Design review of the part built by this model. Coordinates are the model's own, in mm. Face numbers are marked on the shaded views. A direction names the side the tool comes from. Give positions to 0.01 mm unless a question says otherwise; leave off trailing zeros. Loops run counter-clockwise (first coordinate to the right, second up) from the corner with the lowest first, then second, coordinate; pieces in that order, holes last.
from build123d import *

# Parameters (mm, degrees)
EXTRUDE_2_DEPTH       = 5
SKETCH_3_R            = 8
EXTRUDE_3_DEPTH       = 5
SKETCH_4_W            = 60
SKETCH_4_H            = 40
EXTRUDE_4_DEPTH       = 50
SKETCH_5_W            = 70
SKETCH_5_H            = 70
EXTRUDE_5_DEPTH       = 30
SKETCH_6_R            = 2.5
EXTRUDE_6_DEPTH       = 30
EXTRUDE_11_DEPTH      = 0.5
EXTRUDE_11_DEPTH_BACK = 0.5
EXTRUDE_12_DEPTH      = 0.5
EXTRUDE_12_DEPTH_BACK = 0.5
SKETCH_12_W           = 70
SKETCH_12_H           = 70
EXTRUDE_13_DEPTH      = 40
SKETCH_13_W           = 120
SKETCH_13_H           = 120
EXTRUDE_14_DEPTH      = 50


with BuildPart() as part:
    # 草图1 → 凸台-拉伸2 (new body)
    with BuildSketch(Plane.XY):
        with BuildLine():
            ThreePointArc((-110.317541634, 2.5), (-130, 0), (-110.317541634, -2.5))
            Line((-110.317541634, -2.5), (110.317541634, -2.5))
            ThreePointArc((110.317541634, -2.5), (130, 0), (110.317541634, 2.5))
            Line((110.317541634, 2.5), (-110.317541634, 2.5))
        make_face()
    extrude(amount=EXTRUDE_2_DEPTH)

    # 草图3 → 凸台-拉伸3 (add)
    with BuildSketch(Plane.XY.offset(5)):
        with Locations((-120, 0)):
            Circle(SKETCH_3_R)
        with Locations((120, 0)):
            Circle(SKETCH_3_R)
    extrude(amount=EXTRUDE_3_DEPTH)

    # 草图4 → 凸台-拉伸4 (add)
    with BuildSketch(Plane(origin=(0, 0, 0), x_dir=(-1, 0, 0), z_dir=(0, 0, -1))):
        Rectangle(SKETCH_4_W, SKETCH_4_H)
    extrude(amount=EXTRUDE_4_DEPTH)

    # 草图5 → 凸台-拉伸5 (add)
    with BuildSketch(Plane(origin=(0, 0, -50), x_dir=(-1, 0, 0), z_dir=(0, 0, -1))):
        Rectangle(SKETCH_5_W, SKETCH_5_H)
    extrude(amount=EXTRUDE_5_DEPTH)

    # 草图6 → 凸台-拉伸6 (add)
    with BuildSketch(Plane.XY.offset(5)):
        with Locations(Location((0, 0, 0), (0, 0, 270))):
            Circle(SKETCH_6_R)
    extrude(amount=EXTRUDE_6_DEPTH)

    # 草图10 → 凸台-拉伸11 (add, two sides: drawn at the far end of the back side and taken through both)
    with BuildSketch(Plane(origin=(0, 0, 0), x_dir=(-1, 0, 0), z_dir=(0, -1, 0)).offset(-EXTRUDE_11_DEPTH_BACK)):
        with BuildLine():
            Line((179.5, -35), (-180.5, -35))
            ThreePointArc((-180.5, -35), (-0.5, -215), (179.5, -35))
        make_face()
    extrude(amount=EXTRUDE_11_DEPTH + EXTRUDE_11_DEPTH_BACK)

    # 草图11 → 凸台-拉伸12 (add, two sides: drawn at the far end of the back side and taken through both)
    with BuildSketch(Plane.ZY.offset(0.5).offset(-EXTRUDE_12_DEPTH_BACK)):
        with BuildLine():
            Line((35, 180), (35, -180))
            ThreePointArc((35, -180), (215, 0), (35, 180))
        make_face()
    extrude(amount=EXTRUDE_12_DEPTH + EXTRUDE_12_DEPTH_BACK)

    # 草图12 → 凸台-拉伸13 (add)
    with BuildSketch(Plane(origin=(0, 0, -80), x_dir=(-1, 0, 0), z_dir=(0, 0, -1))):
        Rectangle(SKETCH_12_W, SKETCH_12_H)
    extrude(amount=EXTRUDE_13_DEPTH)

    # 草图13 → 凸台-拉伸14 (add)
    with BuildSketch(Plane(origin=(0, 0, -120), x_dir=(-1, 0, 0), z_dir=(0, 0, -1))):
        Rectangle(SKETCH_13_W, SKETCH_13_H)
    extrude(amount=EXTRUDE_14_DEPTH)


solid = part.part
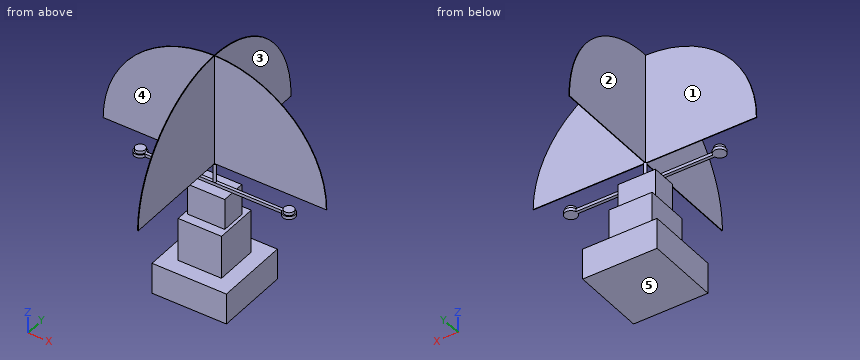
Q1. Take a section at C-C (z = 126). Give the boundary of the cut face in (x, y).
Results:
outline: (-154.8, -0.5) - (-1, -0.5) - (-1, -155.3) - (0, -155.3) - (0, -0.5) - (155.8, -0.5) - (155.8, 0.5) - (0, 0.5) - (0, 155.3) - (-1, 155.3) - (-1, 0.5) - (-154.8, 0.5) - close
Q2. Wall thickness on line 1 (Y direction, x = -124.5, z = 63); line 2 (Z direction, x = -56.5, y = -15.5); line 3 (Y direction, x = -26.5, z = -26): over which ranges is each line inside the solid? List them lowest first.
Results:
line 1: y = -0.5 to 0.5
line 2: z = -170 to -120
line 3: y = -20 to 20
Q3. Take a section at D-D (x = 49). Give the boundary of the cut face in (y, z), plus the area to 3 significant figures.
Results:
outline: (-60, -170) - (60, -170) - (60, -120) - (-60, -120) - close; (-2.5, 0) - (2.5, 0) - (2.5, 5) - (-2.5, 5) - close; (-0.5, 35) - (0.5, 35) - (0.5, 208.34) - (-0.5, 208.34) - close
area: 6,200 mm2
Q4. Tool access review of the marked faces 1, 2, 3, 4 and 5: name each direction out of +Z, -Z, +X, -X, +Y, -Y from which nothing blocks a thin tool from reaching the whole face with its end or side.
Results:
face 1: +Z, -X, +Y
face 2: +Z, -X
face 3: +Z, +X, +Y
face 4: +Z, -X, -Y
face 5: -Z, +X, -X, +Y, -Y
Q5. Insertion check: pin 1 (5 mm diameter, centred on x = 12, z = -116, fed in from -Y); pin 2 (19 mm diameter, centred on x = -3, y = 15, fed in from +Z); pin 3 (1.5 mm diameter, centred on y = 103.5, z = 154.5, fed in from +X); pin 4 (12 mm diameter, centred on x = 21.5, y = -70.5, fed in from +Z). Each pin has a flat end and moves straight along its axis. Give the tip position at first contact, or say it passes through.
Results:
pin 1: stops at y = -35
pin 2: stops at z = 214.91
pin 3: stops at x = 0
pin 4: passes through
Q6. Take a section at B-B (y = -45). Give the boundary of the cut face in (x, z).
Results:
outline: (-60, -170) - (60, -170) - (60, -120) - (-60, -120) - close; (-1, 35) - (0, 35) - (0, 209.28) - (-1, 209.28) - close
Q7. Take a section at A-A (x = -117.5). Give the boundary of the cut face in (y, z), plus the area to 3 significant figures.
Results:
outline: (-9.68, 0) - (9.68, 0) - (9.68, 5) - (7.6, 5) - (7.6, 10) - (-7.6, 10) - (-7.6, 5) - (-9.68, 5) - close; (-0.5, 35) - (0.5, 35) - (0.5, 170.93) - (-0.5, 170.93) - close
area: 309 mm2
